Can you work these out from the model? Positions are in its coordinate system, mm. A direction names the side the tool comes from. Coordinates: 2 decimals unless noted, no trailing zeros. Loops run counter-clockwise (first coordinate to the right, second up) from the corner with the lowest first, then second, coordinate; pieces in that order, holes last. Notation, with made-up numbers: (19, 26) -> (45, 26) arc R14 ccw to (45, 30) -> close; hole circle Ø11 at (-31, 18). An arc over 180 degrees is marked (long way). Use one line per item in the form item = value. Start each with the question number.
(1) Imagine slicing it at A-A (y = 4). List the corners of the cut face in (x, z) for me.
(2) I need wall thicknesses on line 1 (X direction, y = 4.3, z = 62.5); line 2 (Z direction, x = -40.5, y = 6.5); line 3 (Z direction, x = -38.75, y = 4.45). Which ranges of each line are inside material? Lowest first, please. Write a range as [from, to].
(3) Imagine slicing it at C-C (z = 62.5). List the corners of the cut face in (x, y) for me, plus the area to 3 significant figures.
(4) Imagine slicing it at B-B (x = 13). List the corners of the cut face in (y, z) for me.
(5) I'm going to push flat-ended pins straight in: pin 1 (2 mm diameter, centred on y = 4.5, z = 20.5, fed in from -X); pin 2 (4 mm diameter, centred on x = 38.75, z = -62.5, fed in from +Y); pin 3 (1.5 mm diameter, centred on x = 4, y = 4, fed in from +Z); pin 4 (3.5 mm diameter, centred on x = -38.75, z = -62.5, fed in from -Y). Where does each tip first touch, or does it pass through?
(6) Thinking about a two-plate mould opening in Z: for faces 1 (the cylindrical face through (35.977, 4.372, -59.617)), 2 (the flat face through (1, 5, 67.25)), 3 (the flat face through (-43.5, 5, 1)), which applies, released by +Z, released by -Z, zero draft, split by the parting line, or undercut?
(7) Imagine slicing it at D-D (x = 38.75). List the corners of the cut face in (y, z) for me.
(8) On a 3-axis mill with a long thin cutter (end or side, diameter ignored), from which of +Z, -Z, +X, -X, +Y, -Y can I reach the whole of each face in a straight line? I mean faces 4 (the flat face through (-1, 5, -67.25)), 5 (the cylindrical face through (-39.86, 4.43, -63.51)), 6 (the flat face through (1, 0, 1)). Say none if no direction works.
Autodesk Inventor part; units mm, degrees
ref_plane "YZ Plane" through (0, 0, 0) normal (1, 0, 0) x (0, 1, 0)
ref_plane "XZ Plane" through (0, 0, 0) normal (0, 1, 0) x (-1, 0, 0)
ref_plane "XY Plane" through (0, 0, 0) normal (0, 0, 1) x (1, 0, 0)
sketch "Sketch1" plane through (0, 0, 0) normal (0, 1, 0) x (-1, 0, 0)
  line L0 (-45, 68.75) -> (45, 68.75)
  line L1 (45, 68.75) -> (45, -68.75)
  line L2 (45, -68.75) -> (-45, -68.75)
  line L3 (-45, -68.75) -> (-45, 68.75)
  line L4 (-45, 68.75) -> (45, -68.75) construction
  line L5 (45, 68.75) -> (-45, -68.75) construction
  point P0 (0, 0)
  dimension "d0" = 137.5
  dimension "d1" = 90
extrude "Extrusion1" add sketch "Sketch1" along normal blind 8
sketch "Sketch2" plane through (0, 8, 0) normal (0, 1, 0) x (1, 0, 0)
  line L0 (42, -65.75) -> (-42, -65.75)
  line L1 (-42, -65.75) -> (-42, 65.75)
  line L2 (-42, 65.75) -> (42, 65.75)
  line L3 (42, 65.75) -> (42, -65.75)
  line L4 (42, -65.75) -> (-42, 65.75) construction
  line L5 (-42, -65.75) -> (42, 65.75) construction
  point P0 (0, 0)
  dimension "d4" = 131.5
  dimension "d5" = 84
extrude "Extrusion2" cut sketch "Sketch2" against normal blind 1.6
sketch "Sketch3" plane through (0, 6.4, 0) normal (0, 1, 0) x (1, 0, 0)
  line L0 (41, -64.75) -> (-41, -64.75)
  line L1 (-41, -64.75) -> (-41, 64.75)
  line L2 (-41, 64.75) -> (41, 64.75)
  line L3 (41, 64.75) -> (41, -64.75)
  line L4 (41, -64.75) -> (-41, 64.75) construction
  line L5 (-41, -64.75) -> (41, 64.75) construction
  point P0 (0, 0)
  dimension "d8" = 129.5
  dimension "d9" = 82
extrude "Extrusion3" cut sketch "Sketch3" against normal blind 4
sketch "Sketch4" plane through (0, 2.4, 0) normal (0, 1, 0) x (1, 0, 0)
  circle A0 centre (-38.75, -62.5) radius 4
  circle A1 centre (-38.75, 62.5) radius 4
  line L0 (41, -64.75) -> (-41, -64.75)
  circle A2 centre (38.75, -62.5) radius 4
  line L1 (41, 64.75) -> (41, -64.75)
  circle A3 centre (38.75, 62.5) radius 4
  line L2 (-41, -64.75) -> (-41, 64.75)
  point P0 (0, 0)
  point P1 (-41, -59.1928)
  point P2 (-35.4428, -64.75)
  point P3 (41, -59.1928)
  point P4 (35.4428, -64.75)
  dimension "d12" = 8
  dimension "d13" = 8
  dimension "d14" = 125
  dimension "d16" = 2.25
  dimension "d17" = 8
  dimension "d18" = 2.25
  dimension "d19" = 2.25
  dimension "d20" = 77.5
  dimension "d21" = 8
  dimension "d22" = 125
  dimension "d23" = 77.5
  dimension "d24" = 2.25
extrude "Extrusion4" add sketch "Sketch4" along normal blind 4 contours A0 L0 L2 | A3 | A2 L1 L0 | A1 picked at (-37.7393, -61.273) picked at (37.8547, -61.1739)
sketch "Sketch5" plane through (0, 6.4, 0) normal (0, 1, 0) x (1, 0, 0)
  arc A0 (-35.4428, -64.75) -> (-41, -59.1928) centre (-38.75, -62.5) ccw
  circle A1 centre (-38.75, -62.5) radius 1.5
  arc A2 (-41, 59.1928) -> (-35.4428, 64.75) centre (-38.75, 62.5) ccw
  circle A3 centre (-38.75, 62.5) radius 1.5
  arc A4 (35.4428, 64.75) -> (41, 59.1928) centre (38.75, 62.5) ccw
  circle A5 centre (38.75, 62.5) radius 1.5
  arc A6 (41, -59.1928) -> (35.4428, -64.75) centre (38.75, -62.5) ccw
  circle A7 centre (38.75, -62.5) radius 1.5
  point P0 (0, 0)
  dimension "d27" = 3
  dimension "d28" = 3
  dimension "d29" = 3
  dimension "d30" = 3
extrude "Extrusion5" cut sketch "Sketch5" against normal blind 4
fillet "Fillet1" radius 1.5 4 edges at (-42, 7.2, 65.75) (-42, 7.2, -65.75) (42, 7.2, 65.75) (42, 7.2, -65.75)
sketch "Sketch6" plane through (0, 8, 0) normal (0, 1, 0) x (1, 0, 0)
  line L0 (43.5, -67.25) -> (-43.5, -67.25)
  line L1 (-43.5, -67.25) -> (-43.5, 67.25)
  line L2 (-43.5, 67.25) -> (43.5, 67.25)
  line L3 (43.5, 67.25) -> (43.5, -67.25)
  line L4 (43.5, -67.25) -> (-43.5, 67.25) construction
  line L5 (-43.5, -67.25) -> (43.5, 67.25) construction
  line L6 (45.5, -69.25) -> (-45.5, -69.25)
  line L7 (-45.5, -69.25) -> (-45.5, 69.25)
  line L8 (-45.5, 69.25) -> (45.5, 69.25)
  line L9 (45.5, 69.25) -> (45.5, -69.25)
  line L10 (45.5, -69.25) -> (-45.5, 69.25) construction
  line L11 (-45.5, -69.25) -> (45.5, 69.25) construction
  point P0 (0, 0)
  dimension "d35" = 134.5
  dimension "d36" = 87
  dimension "d37" = 138.5
  dimension "d38" = 91
extrude "Extrusion6" cut sketch "Sketch6" against normal blind 6
fillet "Fillet3" radius 1.5 8 edges at (43.5, 5, 67.25) (45, 1, 68.75) (43.5, 5, -67.25) (45, 1, -68.75) (-43.5, 5, -67.25) (-45, 1, -68.75) (-43.5, 5, 67.25) (-45, 1, 68.75)
properties part number "BoardMount"
Worked out:
q1.outline = (-43.5, -65.75) arc R1.5 ccw to (-42, -67.25) -> (42, -67.25) arc R1.5 ccw to (43.5, -65.75) -> (43.5, 65.75) arc R1.5 ccw to (42, 67.25) -> (-42, 67.25) arc R1.5 ccw to (-43.5, 65.75) -> close; hole (-41, -59.19) arc R4 cw to (-35.44, -64.75) -> (35.44, -64.75) arc R4 cw to (41, -59.19) -> (41, 59.19) arc R4 cw to (35.44, 64.75) -> (-35.44, 64.75) arc R4 cw to (-41, 59.19) -> close; hole circle Ø3 at (-38.75, -62.5); hole circle Ø3 at (-38.75, 62.5); hole circle Ø3 at (38.75, -62.5); hole circle Ø3 at (38.75, 62.5)
q2.line_1 = [-43.5, -40.25], [-37.25, -34.75], [34.75, 37.25], [40.25, 43.5]
q2.line_2 = [-67.25, -65.75], [65.75, 67.25]
q2.line_3 = [-67.25, -64], [-61, -58.5], [58.5, 61], [64, 67.25]
q3.outline = (-45, 0) -> (45, 0) -> (45, 2) -> (43.5, 2) -> (43.5, 8) -> (42, 8) -> (42, 6.4) -> (40.25, 6.4) -> (40.25, 2.4) -> (37.25, 2.4) -> (37.25, 6.4) -> (34.75, 6.4) -> (34.75, 2.4) -> (-34.75, 2.4) -> (-34.75, 6.4) -> (-37.25, 6.4) -> (-37.25, 2.4) -> (-40.25, 2.4) -> (-40.25, 6.4) -> (-42, 6.4) -> (-42, 8) -> (-43.5, 8) -> (-43.5, 2) -> (-45, 2) -> close
q3.area = 266 mm2
q4.outline = (0, -68.75) -> (2, -68.75) -> (2, -67.25) -> (8, -67.25) -> (8, -65.75) -> (6.4, -65.75) -> (6.4, -64.75) -> (2.4, -64.75) -> (2.4, 64.75) -> (6.4, 64.75) -> (6.4, 65.75) -> (8, 65.75) -> (8, 67.25) -> (2, 67.25) -> (2, 68.75) -> (0, 68.75) -> close
q5.pin_1 = -43.5
q5.pin_2 = 6.4
q5.pin_3 = 67.25
q5.pin_4 = 0
q6.face_1 = undercut
q6.face_2 = released by +Z
q6.face_3 = zero draft
q7.outline = (0, -68.75) -> (2, -68.75) -> (2, -67.25) -> (8, -67.25) -> (8, -65.75) -> (6.4, -65.75) -> (6.4, -64) -> (2.4, -64) -> (2.4, -61) -> (6.4, -61) -> (6.4, -58.5) -> (2.4, -58.5) -> (2.4, 58.5) -> (6.4, 58.5) -> (6.4, 61) -> (2.4, 61) -> (2.4, 64) -> (6.4, 64) -> (6.4, 65.75) -> (8, 65.75) -> (8, 67.25) -> (2, 67.25) -> (2, 68.75) -> (0, 68.75) -> close
q8.face_4 = -Z, +X, -X, +Y
q8.face_5 = +Y
q8.face_6 = +Z, -Z, +X, -X, -Y
